```python
from build123d import *

# Parameters (mm, degrees)
BOSS_EXTRUDE3_DEPTH = 2.54
BOSS_EXTRUDE4_DEPTH = 2.54
LPATTERN1_COUNT     = 5
LPATTERN1_PITCH     = 2.54
SKETCH8_W           = 100
SKETCH8_H           = 1.5
CUT_EXTRUDE4_DEPTH  = 0.7
BOSS_EXTRUDE5_START = -8.2
SKETCH3_W           = 0.64
SKETCH3_H           = 0.64
BOSS_EXTRUDE5_DEPTH = 11
CHAMFER1_SIZE       = 0.16
CHAMFER1_SIZE2      = 0.5458
CHAMFER2_SIZE       = 0.16
CHAMFER2_SIZE2      = 0.5458
LPATTERN2_START     = 2.22
LPATTERN2_DEPTH     = 0.64
LPATTERN2_START_2   = 4.76
LPATTERN2_2_DEPTH   = 0.64
LPATTERN2_START_3   = 7.3
LPATTERN2_3_DEPTH   = 0.64
LPATTERN2_START_4   = 9.84
LPATTERN2_4_DEPTH   = 0.64
LPATTERN2_START_5   = 12.38
LPATTERN2_5_DEPTH   = 0.64
LPATTERN2_START_6   = -1
LPATTERN2_6_DEPTH   = 2


with BuildPart() as part:
    # Sketch6 → Boss-Extrude3 (new body)
    with BuildSketch(Plane(origin=(0, 0, 0), x_dir=(1, 0, 0), z_dir=(0, 1, 0))):
        Polygon((-1.1825, 0.75), (-1.1825, -0.75), (-0.812519462, -1.25), (0.812519462, -1.25), (1.1825, -0.75), (1.1825, 0.75), (0.812519462, 1.25), (-0.812519462, 1.25), align=None)
    extrude(amount=BOSS_EXTRUDE3_DEPTH)

    # Sketch7 → Boss-Extrude4 (add)
    with BuildSketch(Plane(origin=(0, 0, 0), x_dir=(1, 0, 0), z_dir=(0, 1, 0))):
        Polygon((1.1825, 0.75), (1.1825, -0.75), (1.3825, -0.75), (1.752480538, -1.25), (3.377519462, -1.25), (3.7475, -0.75), (3.7475, 0.75), (3.377519462, 1.25), (1.752480538, 1.25), (1.3825, 0.75), align=None)
    boss_extrude4 = extrude(amount=BOSS_EXTRUDE4_DEPTH)

    # LPattern1: Boss-Extrude4 ×5
    with Locations(*[(i * LPATTERN1_PITCH, 0, 0) for i in range(1, LPATTERN1_COUNT)]):
        add(boss_extrude4)

    # Sketch8 → Cut-Extrude4 (cut)
    with BuildSketch(Plane.XZ):
        with Locations((48.8175, 0)):
            Rectangle(SKETCH8_W, SKETCH8_H)
    extrude(amount=-CUT_EXTRUDE4_DEPTH, mode=Mode.SUBTRACT)

    # Sketch3 → Boss-Extrude5 (add)
    with BuildSketch(Plane(origin=(0, 0, 0), x_dir=(-1, 0, 0), z_dir=(0, -1, 0)).offset(BOSS_EXTRUDE5_START)):
        Rectangle(SKETCH3_W, SKETCH3_H)
    extrude(amount=BOSS_EXTRUDE5_DEPTH)

    # Chamfer1
    chamfer1_edges = [part.edges().sort_by_distance(p)[0] for p in [
        (-0.32, -2.8, 0),
        (0, -2.8, -0.32),
        (0.32, -2.8, 0),
        (0, -2.8, 0.32),
    ]]
    chamfer1_side = [part.faces().sort_by_distance(p)[0] for p in [
        (0, -2.8, 0),
    ]]
    chamfer(chamfer1_edges, length=CHAMFER1_SIZE, length2=CHAMFER1_SIZE2, reference=chamfer1_side[0])

    # Chamfer2
    chamfer2_edges = [part.edges().sort_by_distance(p)[0] for p in [
        (-0.32, 8.2, 0),
        (0, 8.2, 0.32),
        (0.32, 8.2, 0),
        (0, 8.2, -0.32),
    ]]
    chamfer2_side = [part.faces().sort_by_distance(p)[0] for p in [
        (0, 8.2, 0),
    ]]
    chamfer(chamfer2_edges, length=CHAMFER2_SIZE, length2=CHAMFER2_SIZE2, reference=chamfer2_side[0])

    # LPattern2: read off the stored shape, not the designer's step
    # LPattern2 outline → LPattern2 (add)
    with BuildSketch(Plane.YZ.offset(LPATTERN2_START)):
        Polygon((-2.2542, 0.32), (-2.8, 0.16), (-2.8, -0.16), (-2.2542, -0.32), (0.7, -0.32), (0.7, 0.32), align=None)
        Polygon((2.54, 0.32), (2.54, -0.32), (7.6542, -0.32), (8.2, -0.16), (8.2, 0.16), (7.6542, 0.32), align=None)
    extrude(amount=LPATTERN2_DEPTH)

    # LPattern2 2 outline → LPattern2 2 (add)
    with BuildSketch(Plane.YZ.offset(LPATTERN2_START_2)):
        Polygon((-2.2542, 0.32), (-2.8, 0.16), (-2.8, -0.16), (-2.2542, -0.32), (0.7, -0.32), (0.7, 0.32), align=None)
        Polygon((2.54, 0.32), (2.54, -0.32), (7.6542, -0.32), (8.2, -0.16), (8.2, 0.16), (7.6542, 0.32), align=None)
    extrude(amount=LPATTERN2_2_DEPTH)

    # LPattern2 3 outline → LPattern2 3 (add)
    with BuildSketch(Plane.YZ.offset(LPATTERN2_START_3)):
        Polygon((-2.2542, 0.32), (-2.8, 0.16), (-2.8, -0.16), (-2.2542, -0.32), (0.7, -0.32), (0.7, 0.32), align=None)
        Polygon((2.54, 0.32), (2.54, -0.32), (7.6542, -0.32), (8.2, -0.16), (8.2, 0.16), (7.6542, 0.32), align=None)
    extrude(amount=LPATTERN2_3_DEPTH)

    # LPattern2 4 outline → LPattern2 4 (add)
    with BuildSketch(Plane.YZ.offset(LPATTERN2_START_4)):
        Polygon((-2.2542, 0.32), (-2.8, 0.16), (-2.8, -0.16), (-2.2542, -0.32), (0.7, -0.32), (0.7, 0.32), align=None)
        Polygon((2.54, 0.32), (2.54, -0.32), (7.6542, -0.32), (8.2, -0.16), (8.2, 0.16), (7.6542, 0.32), align=None)
    extrude(amount=LPATTERN2_4_DEPTH)

    # LPattern2 5 outline → LPattern2 5 (add)
    with BuildSketch(Plane.YZ.offset(LPATTERN2_START_5)):
        Polygon((-2.2542, 0.32), (-2.8, 0.16), (-2.8, -0.16), (-2.2542, -0.32), (0.7, -0.32), (0.7, 0.32), align=None)
        Polygon((2.54, 0.32), (2.54, -0.32), (7.6542, -0.32), (8.2, -0.16), (8.2, 0.16), (7.6542, 0.32), align=None)
    extrude(amount=LPATTERN2_5_DEPTH)

    # LPattern2 6 outline → LPattern2 6 (cut)
    with BuildSketch(Plane.XY.offset(LPATTERN2_START_6)):
        Polygon((2.86, -2.8), (2.86, -2.2542), (2.7, -2.8), align=None)
        Polygon((2.22, -2.8), (2.38, -2.8), (2.22, -2.2542), align=None)
        Polygon((4.76, -2.8), (4.92, -2.8), (4.76, -2.2542), align=None)
        Polygon((5.4, -2.2542), (5.24, -2.8), (5.4, -2.8), align=None)
        Polygon((7.3, -2.8), (7.46, -2.8), (7.3, -2.2542), align=None)
        Polygon((7.94, -2.2542), (7.78, -2.8), (7.94, -2.8), align=None)
        Polygon((9.84, -2.8), (10, -2.8), (9.84, -2.2542), align=None)
        Polygon((10.48, -2.2542), (10.32, -2.8), (10.48, -2.8), align=None)
        Polygon((12.38, -2.8), (12.54, -2.8), (12.38, -2.2542), align=None)
        Polygon((13.02, -2.2542), (12.86, -2.8), (13.02, -2.8), align=None)
        Polygon((2.22, 7.6542), (2.38, 8.2), (2.22, 8.2), align=None)
        Polygon((2.86, 8.2), (2.7, 8.2), (2.86, 7.6542), align=None)
        Polygon((4.76, 7.6542), (4.92, 8.2), (4.76, 8.2), align=None)
        Polygon((5.24, 8.2), (5.4, 7.6542), (5.4, 8.2), align=None)
        Polygon((7.3, 7.6542), (7.46, 8.2), (7.3, 8.2), align=None)
        Polygon((7.78, 8.2), (7.94, 7.6542), (7.94, 8.2), align=None)
        Polygon((9.84, 7.6542), (10, 8.2), (9.84, 8.2), align=None)
        Polygon((10.32, 8.2), (10.48, 7.6542), (10.48, 8.2), align=None)
        Polygon((12.38, 7.6542), (12.54, 8.2), (12.38, 8.2), align=None)
        Polygon((12.86, 8.2), (13.02, 7.6542), (13.02, 8.2), align=None)
    extrude(amount=LPATTERN2_6_DEPTH, mode=Mode.SUBTRACT)


solid = part.part
```
Design review of the part built by this model. Coordinates are the model's own, in mm. Coordinates: 2 decimals unless noted, no trailing zeros. Order: outer loops, then holes, each group sorted by start corner. A loop starts at its lowest first (then second) coordinate and runs counter-clockwise, first axis right, second up.
1) Clearance check with flat-ended pins moving along their axes: pin 1 (1 mm diameter, centred on x = 5.5, y = 4, fed in from +Z); pin 2 (0.5 mm diameter, centred on y = 5.5, z = 0, fed in from -X); pin 3 (1 mm diameter, centred on x = 1.5, y = 4, fed in from +Z). State where each tip first meets the part, or that it passes through.
2) Take a section at B-B, the plane x = 0. Give the boundary of the cut face in (y, z), and give its area (3 significant figures).
3) Take a section at A-A, the plane y = 4.75. Give the boundary of the cut face in (x, z).
4) Take a section at C-C, the plane z = -1.05. Give the boundary of the cut face in (x, y), and give its area (3 significant figures).
5) Take a section at D-D, the plane x = 2. Give the boundary of the cut face in (y, z), and give its area (3 significant figures).
6) Wall thickness on line 1 along X through (y, z) = (4, -0.05); line 2 along X through (y, z) = (1.5, -0.8); line 3 along Y through (x, z) = (1, 0): over which ranges is each line inside the solid? List them lowest first.
Returned:
1. pin 1: stops at z = 0.32
1. pin 2: stops at x = -0.32
1. pin 3: passes through
2. outline: (-2.8, -0.16) - (-2.25, -0.32) - (0.7, -0.32) - (0.7, -0.75) - (0, -0.75) - (0, -1.25) - (2.54, -1.25) - (2.54, -0.32) - (7.65, -0.32) - (8.2, -0.16) - (8.2, 0.16) - (7.65, 0.32) - (2.54, 0.32) - (2.54, 1.25) - (0, 1.25) - (0, 0.75) - (0.7, 0.75) - (0.7, 0.32) - (-2.25, 0.32) - (-2.8, 0.16) - close
2. area: 11.0 mm2
3. outline: (-0.32, -0.32) - (0.32, -0.32) - (0.32, 0.32) - (-0.32, 0.32) - close; (2.22, -0.32) - (2.86, -0.32) - (2.86, 0.32) - (2.22, 0.32) - close; (4.76, -0.32) - (5.4, -0.32) - (5.4, 0.32) - (4.76, 0.32) - close; (7.3, -0.32) - (7.94, -0.32) - (7.94, 0.32) - (7.3, 0.32) - close; (9.84, -0.32) - (10.48, -0.32) - (10.48, 0.32) - (9.84, 0.32) - close; (12.38, -0.32) - (13.02, -0.32) - (13.02, 0.32) - (12.38, 0.32) - close
4. outline: (-0.96, 0) - (0.96, 0) - (0.96, 2.54) - (-0.96, 2.54) - close; (1.6, 0) - (3.53, 0) - (3.53, 2.54) - (1.6, 2.54) - close; (4.14, 0) - (6.07, 0) - (6.07, 2.54) - (4.14, 2.54) - close; (6.68, 0) - (8.61, 0) - (8.61, 2.54) - (6.68, 2.54) - close; (9.22, 0) - (11.15, 0) - (11.15, 2.54) - (9.22, 2.54) - close; (11.76, 0) - (13.69, 0) - (13.69, 2.54) - (11.76, 2.54) - close
4. area: 29.3 mm2
5. outline: (0, -1.25) - (2.54, -1.25) - (2.54, 1.25) - (0, 1.25) - (0, 0.75) - (0.7, 0.75) - (0.7, -0.75) - (0, -0.75) - close
5. area: 5.30 mm2
6. line 1: x = -0.32 to 0.32, 2.22 to 2.86, 4.76 to 5.4, 7.3 to 7.94, 9.84 to 10.48, 12.38 to 13.02
6. line 2: x = -1.15 to 1.15, 1.42 to 3.71, 3.96 to 6.25, 6.5 to 8.79, 9.04 to 11.33, 11.58 to 13.87
6. line 3: y = 0.7 to 2.54
